```python
from build123d import *

# Parameters (mm, degrees)
SKETCH_4_W          = 90
SKETCH_4_H          = 60
EXTRUDE_1_DEPTH     = 70
SKETCH_5_W          = 60
SKETCH_5_H          = 40
CUT_EXTRUDE_1_DEPTH = 70
SKETCH_6_R          = 9
CUT_EXTRUDE_2_DEPTH = 9
FILLET_1_R          = 20


with BuildPart() as part:
    # 스케치4 → 보스-돌출1 (new body)
    with BuildSketch(Plane.XY):
        with Locations((45, 30)):
            Rectangle(SKETCH_4_W, SKETCH_4_H)
    extrude(amount=EXTRUDE_1_DEPTH)

    # 스케치5 → 컷-돌출1 (cut)
    with BuildSketch(Plane.XY.offset(70)):
        with Locations((60, 40)):
            Rectangle(SKETCH_5_W, SKETCH_5_H)
    extrude(amount=-CUT_EXTRUDE_1_DEPTH, mode=Mode.SUBTRACT)

    # 스케치6 → 컷-돌출2 (cut)
    with BuildSketch(Plane(origin=(0, 60, 0), x_dir=(1, 0, 0), z_dir=(0, 1, 0))):
        with Locations((15, -35)):
            Circle(SKETCH_6_R)
    extrude(amount=-CUT_EXTRUDE_2_DEPTH, mode=Mode.SUBTRACT)

    # 필렛1
    fillet_1_edges = [part.edges().sort_by_distance(p)[0] for p in [
        (90, 10, 70),
        (90, 10, 0),
    ]]
    fillet(fillet_1_edges, radius=FILLET_1_R)


solid = part.part
```
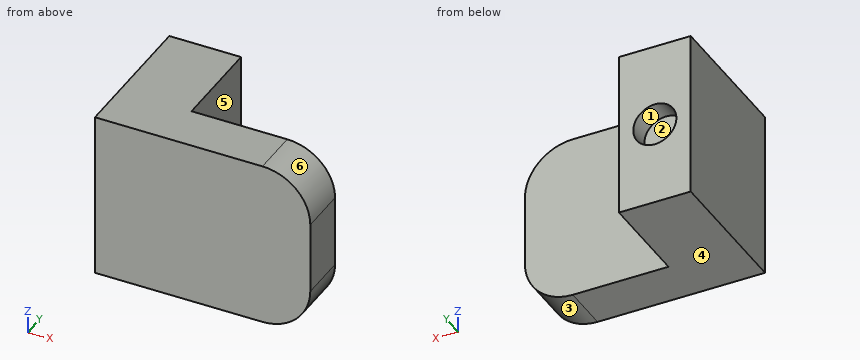
Can you work these out from the model? Positions are in its coordinate system, mm. Face numbers are marked on the shaded views. A direction names the side the tool comes from. Round coordinates to 2 decimals unless told otherwise and drop trailing zeros. Order: outer loops, then holes, each group sorted by start corner. A loop starts at its lowest first (then second) coordinate and runs counter-clockwise, first axis right, second up. Notation, with made-up numbers: (84.5, -23) -> (88.5, -23) arc R12 ccw to (88.5, -11) -> close; hole circle Ø4 at (42.5, 67.5). An arc over 180 degrees is marked (long way). Return JSON: item names as keys, results as strings. Group by question number.
1. I need wall thicknesses on line 1 (X direction, y = 53, z = 35); line 2 (Z direction, x = 15, y = 57); line 3 (X direction, y = 4, z = 19.5). Which ranges of each line are inside material? Lowest first, please. Write a range as [from, to].
2. If we section it at D-D, the plane y = 44.5: Write out the boundary of the cut face in (x, z).
3. If we section it at B-B, the plane x = 15: Write out the boundary of the cut face in (y, z), then the cut area to 3 significant figures.
4. Which directions (+Z, -Z, +X, -X, +Y, -Y) give clear straight access to the entire face, cutting with the end or side of a thin tool? Please do the marked faces 5 and 6.
5. We'd pull the mould along X, two halves only. Please class the marked faces 1, 2, 3 and 4: released by +X, released by -X, zero draft, split by the parting line, or undercut.
6. If we section it at C-C, the plane y = 53: Write out the boundary of the cut face in (x, z), then the cut area to 3 significant figures.
7. If we section it at A-A, the plane z = 35: Write out the boundary of the cut face in (x, y), then the cut area to 3 significant figures.
8. Will these pins go through, and if not, where does the flat tip stop? pin 1 (20 mm diameter, centred on x = 19.5, z = 37, fed in from +Y); pin 2 (20 mm diameter, centred on y = 36.5, z = 44, fed in from +X); pin 3 (10 mm diameter, centred on x = 47.5, z = 8.5, fed in from +Y); pin 4 (4 mm diameter, centred on x = 16.5, z = 35.5, fed in from +Y).
Output values:
{
 "1": {"line 1": "[0, 6], [24, 30]", "line 2": "[0, 26], [44, 70]", "line 3": "[0, 89.99]"},
 "2": {"outline": "(0, 0) -> (30, 0) -> (30, 70) -> (0, 70) -> close"},
 "3": {"outline": "(0, 0) -> (60, 0) -> (60, 26) -> (51, 26) -> (51, 44) -> (60, 44) -> (60, 70) -> (0, 70) -> close", "area": "4,040 mm²"},
 "4": {"face 5": "+Z, -Z, +X, +Y", "face 6": "+Z, +X, +Y, -Y"},
 "5": {"face 1": "undercut", "face 2": "undercut", "face 3": "released by +X", "face 4": "zero draft"},
 "6": {"outline": "(0, 0) -> (30, 0) -> (30, 70) -> (0, 70) -> close; hole circle Ø18 at (15, 35)", "area": "1,850 mm²"},
 "7": {"outline": "(0, 0) -> (90, 0) -> (90, 20) -> (30, 20) -> (30, 60) -> (24, 60) -> (24, 51) -> (6, 51) -> (6, 60) -> (0, 60) -> close", "area": "2,840 mm²"},
 "8": {"pin 1": "y = 60", "pin 2": "x = 30", "pin 3": "y = 20", "pin 4": "y = 51"}
}
